Geometry check sheet. Reference: the model listing, model coordinates, mm. Face numbers are marked on the shaded views. A direction names the side the tool comes from. Give positions to 0.01 mm unless a question says otherwise; leave off trailing zeros. Loops run counter-clockwise (first coordinate to the right, second up) from the corner with the lowest first, then second, coordinate; pieces in that order, holes last. Notation, with made-up numbers: (32, -10) -> (72, -10) arc R15 ccw to (72, -4) -> close; hole circle Ø4 at (-35.5, 77). An arc over 180 degrees is marked (long way). Write item = value, one per line. Start each with the question number.
Autodesk Inventor part; units mm, degrees
ref_plane "YZ Plane" through (0, 0, 0) normal (1, 0, 0) x (0, 1, 0)
ref_plane "XZ Plane" through (0, 0, 0) normal (0, 1, 0) x (-1, 0, 0)
ref_plane "XY Plane" through (0, 0, 0) normal (0, 0, 1) x (1, 0, 0)
sketch "スケッチ1" plane through (0, 0, 0) normal (1, 0, 0) x (0, 1, 0)
  line L0 (0, 0) -> (1.25, 0)
  line L1 (1.25, 0) -> (1.25, -6)
  line L2 (1.25, -6) -> (0, -6)
  line L3 (0, -6) -> (0, 0)
  line L4 (0, -6) -> (2.25, -6)
  line L5 (2.25, -6) -> (2.25, -8)
  line L6 (2.25, -8) -> (0, -8)
  line L7 (0, -8) -> (0, -6)
  line L8 (2.25, -7.8) -> (2.05, -8)
  line L9 (1.25, -0.12) -> (1.13, 0)
  point P0 (2.25, -7)
  dimension "d0" = 45
  dimension "d1" = 2.25
  dimension "d2" = 2
  dimension "d3" = 6
  dimension "d7" = 1.25
  dimension "d10" = 45
  dimension "d11" = 0.2
  dimension "d12" = 0.12
revolve "回転1" add sketch "スケッチ1" angle 360 about axis through (0, 0, -6) along (0, 0, 1) contours L0 L9 L1 L2 L3 | L2 L4 L5 L8 L6 L7
thread "ねじ2"
properties part number "CSH-316L-M2-5" material "ステンレス鋼"
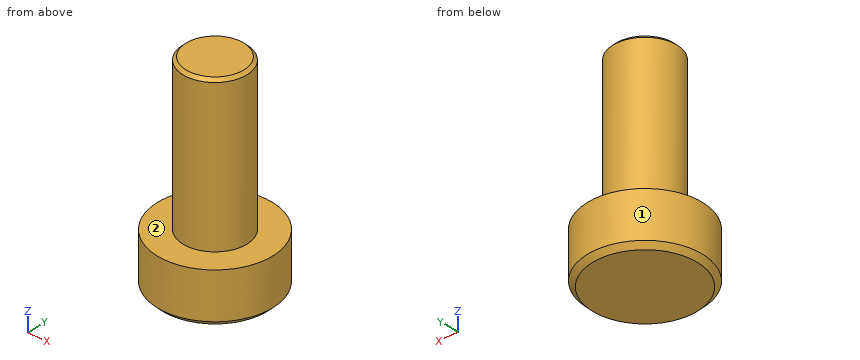
1) Thickness scan on line 1 (Z direction, x = 0.65, y = -1.7); line 2 (Y direction, x = 0, z = -4.5); line 3 (X direction, y = -1, z = -7). Record the ranges inside material, lowest first.
2) Section check D-D (z = -4.75). Enter the section's corners in (x, y), plus the area to 3 significant figures.
3) Tool access check on the marked faces 1 and 2. Record the directions out of +Z, -Z, +X, -X, +Y, -Y that give a thin tool (end or side, any length) a straight path to the whole face; none if there is none.
4) Section check C-C (z = -7). Enter the section's corners in (x, y), plus the area to 3 significant figures.
5) Depth check by flat-ended pin: pin 1 Ø1.5 at (y, z) = (-1.5, -4) entering from -X. Enter the tip coordinate at first touch or a pass-through.
6) Section check A-A (y = 0). Enter the section's corners in (x, z), plus the area to 3 significant figures.
Check result:
q1.line_1 = -8 to -6
q1.line_2 = -1.25 to 1.25
q1.line_3 = -2.02 to 2.02
q2.outline = circle Ø2.5 at (0, 0)
q2.area = 4.91 mm2
q3.face_1 = +Z, -Z
q3.face_2 = +Z
q4.outline = circle Ø4.5 at (0, 0)
q4.area = 15.9 mm2
q5.pin_1 = -1
q6.outline = (-2.25, -7.8) -> (-2.05, -8) -> (2.05, -8) -> (2.25, -7.8) -> (2.25, -6) -> (1.25, -6) -> (1.25, -0.12) -> (1.13, 0) -> (-1.13, 0) -> (-1.25, -0.12) -> (-1.25, -6) -> (-2.25, -6) -> close
q6.area = 23.9 mm2
